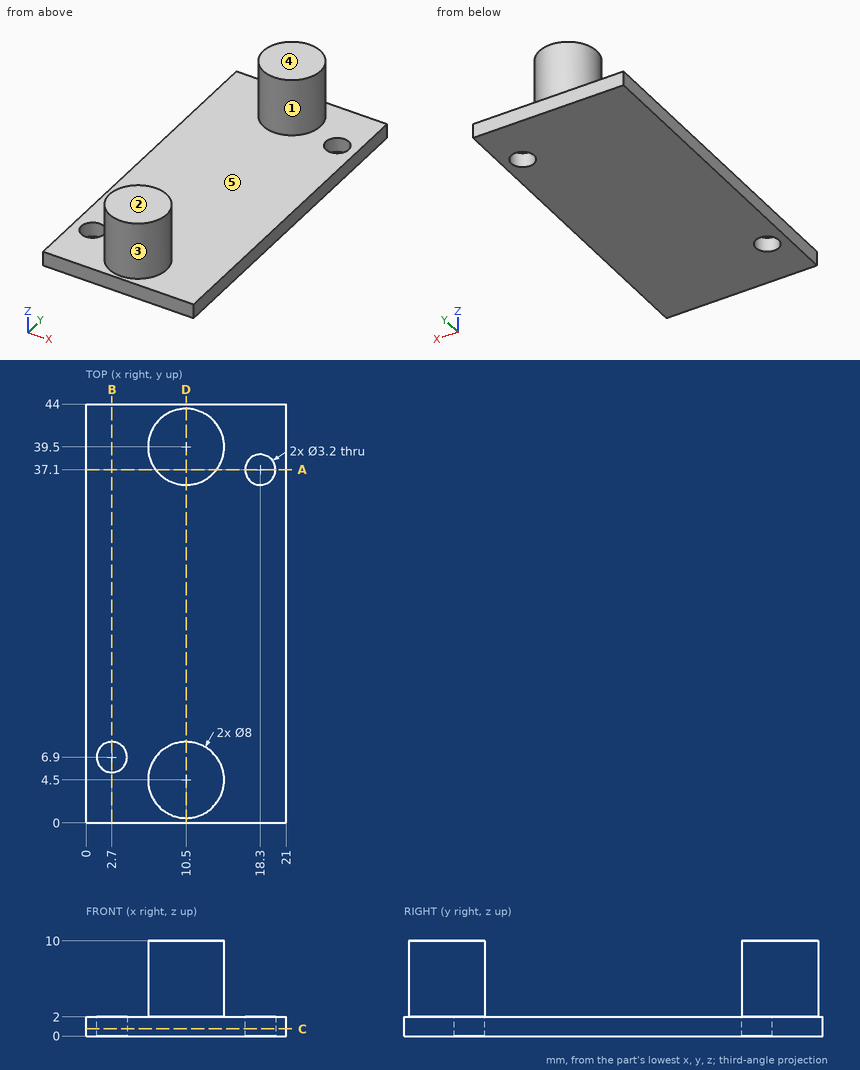
Geometry: see drawing. Coordinates: mm, zero at the bounding-box minimum. A direction names the side the tool comes from. Give positions to 0.01 mm unless a question says otherwise; leave off trailing zeros. Loops run counter-clockwise (first coordinate to the right, second up) from the corner with the lowest first, then second, coordinate; pieces in that order, holes last. Notation, with made-up numbers: (18.5, 44) -> (39.5, 44) arc R17 cw to (39.5, 72) -> close; hole circle Ø11 at (33, 57). An arc over 180 degrees is marked (long way). Put each result on its own line as item: value.
1. Ray query, line 1 along Y through (x, z) = (2.7, 0.8); line 2 along Y through (x, z) = (18.3, 1.65); line 3 along Z through (x, y) = (13.5, 8). Return the intervals inside material, ascending. Write a range as [from, to].
Taken from the geometry:
line 1: y = [0, 5.3], [8.5, 44]
line 2: y = [0, 35.5], [38.7, 44]
line 3: z = [0, 2]
2. Cut plane D-D (x = 10.5). Return the cut outline in (y, z), plus the area to 3 significant figures.
Taken from the geometry:
outline: (0, 0) -> (44, 0) -> (44, 2) -> (43.5, 2) -> (43.5, 10) -> (35.5, 10) -> (35.5, 2) -> (8.5, 2) -> (8.5, 10) -> (0.5, 10) -> (0.5, 2) -> (0, 2) -> close
area: 216 mm2
3. Cut plane C-C (z = 0.75). Return the cut outline in (x, y).
Taken from the geometry:
outline: (0, 0) -> (21, 0) -> (21, 44) -> (0, 44) -> close; hole circle Ø3.2 at (2.7, 6.9); hole circle Ø3.2 at (18.3, 37.1)
4. Pull-direction query (Y, two-part tool) for the marked faces 3, 4 and 5; classes: released by +Y, released by -Y, zero draft, split by the parting line, or undercut.
Taken from the geometry:
face 3: undercut
face 4: zero draft
face 5: undercut
5. Set-up query: the marked faces 1 and 2. Return all of +Z, -Z, +X, -X, +Y, -Y with unobstructed straight access to the full face (end or side cutting, diameter ignored); none if empty.
Taken from the geometry:
face 1: +Z
face 2: +Z, +X, -X, +Y, -Y
6. Pin query (flat end, axial travel): P1, Ø3, axis at x = 18.3, y = 37.1, coming from the +Z side; P2, Ø2, axis at x = 15.5, y = 29, coming from the +Z side. Return the tip coordinate at first contact, or that it passes through.
Taken from the geometry:
P1: passes through
P2: stops at z = 2
7. Cut plane A-A (y = 37.1). Return the cut outline in (x, z).
Taken from the geometry:
outline: (0, 0) -> (16.7, 0) -> (16.7, 2) -> (13.7, 2) -> (13.7, 10) -> (7.3, 10) -> (7.3, 2) -> (0, 2) -> close; (19.9, 0) -> (21, 0) -> (21, 2) -> (19.9, 2) -> close
8. Cut plane B-B (x = 2.7). Return the cut outline in (y, z).
Taken from the geometry:
outline: (0, 0) -> (5.3, 0) -> (5.3, 2) -> (0, 2) -> close; (8.5, 0) -> (44, 0) -> (44, 2) -> (8.5, 2) -> close
